Autodesk Inventor part; units mm, degrees
ref_plane "YZ Plane" through (0, 0, 0) normal (1, 0, 0) x (0, 1, 0)
ref_plane "XZ Plane" through (0, 0, 0) normal (0, 1, 0) x (-1, 0, 0)
ref_plane "XY Plane" through (0, 0, 0) normal (0, 0, 1) x (1, 0, 0)
sketch "スケッチ1" plane through (0, 0, 0) normal (0, 0, 1) x (1, 0, 0)
  circle A0 centre (0, 0) radius 21
  dimension "d0" = 42
extrude "押し出し1" add sketch "スケッチ1" along normal blind 39.2
sketch "スケッチ2" plane through (0, 0, 39.2) normal (0, 0, 1) x (1, 0, 0)
  circle A0 centre (0, 0) radius 12.5
  dimension "d3" = 25
extrude "押し出し2" add sketch "スケッチ2" along normal blind 2
sketch "スケッチ3" plane through (0, 0, 41.2) normal (0, 0, 1) x (1, 0, 0)
  circle A0 centre (0, 0) radius 4
  dimension "d6" = 8
extrude "押し出し3" add sketch "スケッチ3" along normal blind 20
sketch "スケッチ4" plane through (0, 0, 61.2) normal (0, 0, 1) x (1, 0, 0)
  circle A0 centre (0, 0) radius 4
  circle A1 centre (0, 0) radius 4
  line L0 (-2.6458, 3) -> (2.6458, 3)
  point P0 (0, 3)
  dimension "d9" = 3
extrude "押し出し4" cut sketch "スケッチ4" against normal blind 12 contours L0 A0 picked at (-0.6179, 3.1815)
sketch "スケッチ5" plane through (0, 0, 41.2) normal (0, 0, 1) x (1, 0, 0)
  circle A0 centre (0, 0) radius 12.5
  line L0 (-11.5, 4.899) -> (-11.5, -4.899)
  line L1 (11.5, -4.899) -> (11.5, 4.899)
  point P0 (-11.5, 0)
  point P1 (11.5, 0)
  dimension "d12" = 11.5
  dimension "d13" = 11.5
extrude "押し出し5" cut sketch "スケッチ5" against normal blind 2 contours A0 L1 | L0 A0
equation "\"BendRadius\" = Thickness"
equation "\"BendReliefWidth\" = Thickness"
equation "\"BendReliefDepth\" = 0.5 * Thickness"
equation "\"CornerReliefSize\" = 4 * Thickness"
equation "\"MinimumRemnant\" = 2 * Thickness"
equation "\"TransitionRadius\" = BendRadius"
equation "\"JacobiRadiusSize\" = BendRadius"
equation "\"GapSize\" = Thickness"
properties part number "nhk_purry" material "ステンレス鋼"
Can you work these out from the model? Positions are in its coordinate system, mm. A direction names the side the tool comes from. Give positions to 0.01 mm unless a question says otherwise; leave off trailing zeros. Order: outer loops, then holes, each group sorted by start corner. A loop starts at its lowest first (then second) coordinate and runs counter-clockwise, first axis right, second up. Notation, with made-up numbers: M 61,12.25 L 110,12.25 A21 cw 110,44.25 Z; hole C 48,86 d7. An arc over 180 degrees is marked long. One line per item, written item: value.
1) I want a section at C-C, the plane z = 21. List the corners of the cut face in (x, y) for me, plus the area to 3 significant figures.
Answer sheet:
outline: C 0,0 d42
area: 1,390 mm^2
2) I want a section at A-A, the plane x = 0. List the corners of the cut face in (y, z) for me, plus the area to 3 significant figures.
Answer sheet:
outline: M -21,0 L 21,0 L 21,39.2 L 12.5,39.2 L 12.5,41.2 L 4,41.2 L 4,49.2 L 3,49.2 L 3,61.2 L -4,61.2 L -4,41.2 L -12.5,41.2 L -12.5,39.2 L -21,39.2 Z
area: 1,840 mm^2
3) For P1, Ø4, axis at x = 0, z = 54.5, coming from the +Y side; P2, Ø2, axis at x = -10, y = -2.5, coming from the +Z side; P3, Ø3, axis at x = 4, z = 42, coming from the -Y side, each with a flat end and sliding along its axis, tell me the tip position at first contact or that it passes through.
Answer sheet:
P1: stops at y = 3
P2: stops at z = 41.2
P3: stops at y = -12.2
4) I want a section at D-D, the plane y = -7. List the corners of the cut face in (x, z) for me, plus the area to 3 significant figures.
Answer sheet:
outline: M -19.8,0 L 19.8,0 L 19.8,39.2 L 10.36,39.2 L 10.36,41.2 L -10.36,41.2 L -10.36,39.2 L -19.8,39.2 Z
area: 1,590 mm^2
5) I want a section at B-B, the plane y = 0. List the corners of the cut face in (x, z) for me.
Answer sheet:
outline: M -21,0 L 21,0 L 21,39.2 L 11.5,39.2 L 11.5,41.2 L 4,41.2 L 4,61.2 L -4,61.2 L -4,41.2 L -11.5,41.2 L -11.5,39.2 L -21,39.2 Z
6) Please list where these lines run through material, in increasing order: line 1 along Z through (x, y) = (-14, -4); line 2 along Z through (x, y) = (-4, -6.5); line 3 along Y through (x, z) = (1, 31).
Answer sheet:
line 1: z = 0 to 39.2
line 2: z = 0 to 41.2
line 3: y = -20.98 to 20.98
7) On a 3-axis mill with a long thin cutter (end or side, diameter ignored), from which of +Z, -Z, +X, -X, +Y, -Y can I reach the whole of each face in a straight line? I mean faces 1 (the face through (9, -9, 39.2)), 2 (the face through (-0.2, 12.5, 40.2)), 3 (the face through (11.5, 0, 40)), 4 (the face through (0.2, -12.5, 40.2)), 5 (the face through (0, 3, 55)). Say none if no direction works.
Answer sheet:
face 1: +Z
face 2: +Z, +Y
face 3: +Z, +X, +Y, -Y
face 4: +Z, -Y
face 5: +Z, +X, -X, +Y
